from build123d import *
from OCP.BRepFilletAPI import BRepFilletAPI_MakeChamfer

# Parameters (mm, degrees)
SKETCH1_R           = 152.4
BOSS_EXTRUDE1_DEPTH = 6.35
SKETCH2_R           = 2.413
CUT_EXTRUDE1_DEPTH  = 10.16
SKETCH4_R           = 2.413
CUT_EXTRUDE2_DEPTH  = 7.62
CHAMFER1_SIZE       = 2.54
CHAMFER1_SIZE2      = 2.207988314
SKETCH6_R           = 152.4
SKETCH6_R_2         = 127
CUT_EXTRUDE3_DEPTH  = 7.62
SKETCH7_R           = 3.175
CUT_EXTRUDE4_DEPTH  = 15.24


with BuildPart() as part:
    # Sketch1 → Boss-Extrude1 (new body)
    with BuildSketch(Plane.XY):
        Circle(SKETCH1_R)
        with BuildLine():
            ThreePointArc((-5e-08, 34.925), (34.925, -5.6e-08), (-1.61e-07, -34.925))
            Line((-1.61e-07, -34.925), (-50.8, -34.925))
            ThreePointArc((-50.8, -34.925), (-85.725, 0), (-50.8, 34.925))
            Line((-50.8, 34.925), (-5e-08, 34.925))
        make_face(mode=Mode.SUBTRACT)
    extrude(amount=BOSS_EXTRUDE1_DEPTH)

    # Sketch2 → Cut-Extrude1 (cut)
    with BuildSketch(Plane(origin=(0, 0, 0), x_dir=(-1, 0, 0), z_dir=(0, 0, -1))):
        with Locations((111.125, 20.6375)):
            Circle(SKETCH2_R)
        with Locations((111.125, 0)):
            Circle(SKETCH2_R)
        with Locations((111.125, -20.6375)):
            Circle(SKETCH2_R)
    extrude(amount=-CUT_EXTRUDE1_DEPTH, mode=Mode.SUBTRACT)

    # Sketch4 → Cut-Extrude2 (cut)
    with BuildSketch(Plane.XY.offset(6.35)):
        with Locations((61.8998, 20.6375)):
            Circle(SKETCH4_R)
        with Locations((61.8998, 0)):
            Circle(SKETCH4_R)
        with Locations((61.8998, -20.6375)):
            Circle(SKETCH4_R)
    extrude(amount=-CUT_EXTRUDE2_DEPTH, mode=Mode.SUBTRACT)

    # Chamfer1: one chamfer whose edges measure the first distance from different faces: ONE call of the kernel's chamfer builder (chamfer() names one face for all edges)
    chamfer1_edges_1 = [part.edges().sort_by_distance(p)[0] for p in [
        (-108.712, 20.6375, 0),
        (-108.712, 0, 0),
        (-108.712, -20.6375, 0),
    ]]
    chamfer1_side_1 = [part.faces().sort_by_distance(p)[0] for p in [
        (-148.089477062, 0, 0),
    ]]
    chamfer1_edges_2 = [part.edges().sort_by_distance(p)[0] for p in [
        (59.4868, 20.6375, 0),
    ]]
    chamfer1_side_2 = [part.faces().sort_by_distance(p)[0] for p in [
        (59.4868, 20.6375, 3.175),
    ]]
    chamfer1_edges_3 = [part.edges().sort_by_distance(p)[0] for p in [
        (59.4868, 0, 0),
    ]]
    chamfer1_side_3 = [part.faces().sort_by_distance(p)[0] for p in [
        (59.4868, 0, 3.175),
    ]]
    chamfer1_edges_4 = [part.edges().sort_by_distance(p)[0] for p in [
        (59.4868, -20.6375, 0),
    ]]
    chamfer1_side_4 = [part.faces().sort_by_distance(p)[0] for p in [
        (59.4868, -20.6375, 3.175),
    ]]
    chamfer1 = BRepFilletAPI_MakeChamfer(part.part.solid().wrapped)
    for e in chamfer1_edges_1:
        chamfer1.Add(CHAMFER1_SIZE, CHAMFER1_SIZE2, e.wrapped, chamfer1_side_1[0].wrapped)  # the first distance lies on this face
    for e in chamfer1_edges_2:
        chamfer1.Add(CHAMFER1_SIZE, CHAMFER1_SIZE2, e.wrapped, chamfer1_side_2[0].wrapped)  # the first distance lies on this face
    for e in chamfer1_edges_3:
        chamfer1.Add(CHAMFER1_SIZE, CHAMFER1_SIZE2, e.wrapped, chamfer1_side_3[0].wrapped)  # the first distance lies on this face
    for e in chamfer1_edges_4:
        chamfer1.Add(CHAMFER1_SIZE, CHAMFER1_SIZE2, e.wrapped, chamfer1_side_4[0].wrapped)  # the first distance lies on this face
    add(Compound.cast(chamfer1.Shape()), mode=Mode.REPLACE)

    # Sketch6 → Cut-Extrude3 (cut)
    with BuildSketch(Plane(origin=(0, 0, 0), x_dir=(-1, 0, 0), z_dir=(0, 0, -1))):
        Circle(SKETCH6_R)
        Circle(SKETCH6_R_2, mode=Mode.SUBTRACT)
    extrude(amount=-CUT_EXTRUDE3_DEPTH, mode=Mode.SUBTRACT)

    # Sketch5 → Revolve1 (revolve)
    with BuildSketch(Plane(origin=(0, 0, 0), x_dir=(1, 0, 0), z_dir=(0, 1, 0))):
        Polygon((-127, -6.35), (-127, 0), (-130.175, -3.175), align=None)
    revolve(axis=Axis((0, 0, 0), (0, 0, 1)))

    # Sketch7 → Cut-Extrude4 (cut)
    with BuildSketch(Plane(origin=(0, 0, 0), x_dir=(-1, 0, 0), z_dir=(0, 0, -1))):
        with Locations((40.095656626, 96.799478019)):
            Circle(SKETCH7_R)
        with Locations((96.799478019, 40.095656626)):
            Circle(SKETCH7_R)
        with Locations((96.799478019, -40.095656626)):
            Circle(SKETCH7_R)
        with Locations((40.095656626, -96.799478019)):
            Circle(SKETCH7_R)
        with Locations((-40.095656626, -96.799478019)):
            Circle(SKETCH7_R)
        with Locations((-96.799478019, -40.095656626)):
            Circle(SKETCH7_R)
        with Locations((-96.799478019, 40.095656626)):
            Circle(SKETCH7_R)
        with Locations((-40.095656626, 96.799478019)):
            Circle(SKETCH7_R)
    extrude(amount=-CUT_EXTRUDE4_DEPTH, mode=Mode.SUBTRACT)


solid = part.part
The listing builds one solid part. Answer for the finished solid, in the listing's coordinates (mm). A direction names the side the tool comes from. Coordinates: 2 decimals unless noted, no trailing zeros. Answer in a Markdown table with one row per item. Add a question column.
1. Consider line 1 (X direction, y = -38.5, z = 5); line 2 (Y direction, x = 98, z = 5.75); line 3 (X direction, y = -39, z = 4.75). Determine where each line is inside the solid, lowest interval first. Write a range as [from, to].
2. For faces 1 (the conical face through (-113.47, -0.97, 2.1)), 2 (the cylindrical face through (-85.717, -0.768, 3.131)), determine the directions among +Z, -Z, +X, -X, +Y, -Y from which every point of the face is accessible in a straight line to the end or side of a thin tool.
3. A flat-ended cylindrical pin translates along its axis: P1, Ø3, axis at x = -28, z = 4.5, coming from the -Y side. Find the tip coordinate at first contact, or state that the pin passes through.
4. The part is cut by section A-A, the plane z = 5. Count the separate pieces of the cut face and the enclosed holes in it, then the cut area to 3 significant figures.
5. Determine the mould class of faces 3 (the cylindrical face through (-96.111, -43.195, 3.131)), 4 (the flat face through (-25, -34.925, 3)), 5 (the flat face through (26, -26, 0)) for opening direction Y: +Y half, -Y half, draft (parallel to the pull), parting line (faces both ways), or undercut.
Answer below:
| question | item | result |
|---|---|---|
| 1 | line 1 | [-122.44, -99.54], [-94.05, 94.05], [99.54, 122.44] |
| 1 | line 2 | [-81.72, -43.03], [-37.16, 37.16], [43.03, 81.72] |
| 1 | line 3 | [-122.54, -99.78], [-93.82, 93.82], [99.78, 122.54] |
| 2 | face 1 | -Z |
| 2 | face 2 | +Z, -Z |
| 3 | P1 | y = -127.28 |
| 4 | separate pieces | 1 |
| 4 | enclosed holes | 15 |
| 4 | area | 44,000 mm2 |
| 5 | face 3 | undercut |
| 5 | face 4 | undercut |
| 5 | face 5 | draft |
